Here's how the part is built. I have some questions about the finished solid (model axes, mm). Round coordinates to 2 decimals unless told otherwise and drop trailing zeros. Order: outer loops, then holes, each group sorted by start corner. A loop starts at its lowest first (then second) coordinate and runs counter-clockwise, first axis right, second up.
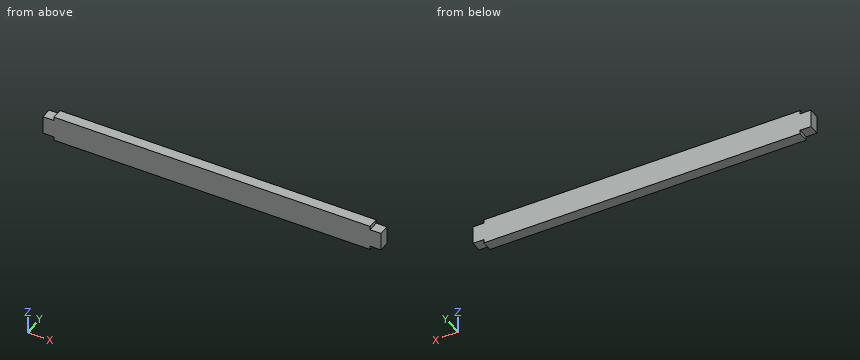
```python
from build123d import *

# Parameters (mm, degrees)
F0_W     = 38.1
F0_H     = 88.9
F1_DEPTH = 1117.6
F2_W     = 38.1
F2_H     = 63.5
F3_DEPTH = 38.1
F4_W     = 38.1
F4_H     = 63.5
F5_DEPTH = 38.1


with BuildPart() as f1:
    # F0 (on Right) → F1 (new body)
    with BuildSketch(Plane.YZ):
        with Locations((19.05, 44.45)):
            Rectangle(F0_W, F0_H)
    extrude(amount=-F1_DEPTH)

    # F2 (on face) → F3 (join)
    with BuildSketch(Plane.YZ):
        with Locations((19.05, 44.45)):
            Rectangle(F2_W, F2_H)
    extrude(amount=F3_DEPTH)

    # F4 (on face) → F5 (join)
    with BuildSketch(Plane(origin=(-1117.6, 0, 0), x_dir=(0, -1, 0), z_dir=(-1, 0, 0))):
        with Locations((-19.05, 44.45)):
            Rectangle(F4_W, F4_H)
    extrude(amount=F5_DEPTH)


solid = f1.part
```
1. If we section it at A-A, the plane y = 8: Write out the boundary of the cut face in (x, z), and give its area (3 significant figures).
Evaluation:
outline: (-1155.7, 12.7) - (-1117.6, 12.7) - (-1117.6, 0) - (0, 0) - (0, 12.7) - (38.1, 12.7) - (38.1, 76.2) - (0, 76.2) - (0, 88.9) - (-1117.6, 88.9) - (-1117.6, 76.2) - (-1155.7, 76.2) - close
area: 104,000 mm2
2. I'm going to push flat-ended pins straight in: P1, Ø14, axis at y = 24.5, z = 83.5, coming from the -X side; P2, Ø19, axis at x = 11.5, y = 18, coming from the -Z side; P3, Ø4, axis at y = 13.5, z = 6, coming from the +X side. Where does each tip first touch, or does it pass through?
Evaluation:
P1: stops at x = -1117.6
P2: stops at z = 12.7
P3: stops at x = 0
3. I need wall thicknesses on probe 1 along X at (y, z) = (8.5, 10). Which ranges of the line are inside material? Lowest first, please.
Evaluation:
probe 1: x = -1117.6 to 0
